Can you work these out from the model? Positions are in its coordinate system, mm. Give positions to 0.01 mm unless a question says otherwise; leave off trailing zeros. Loops run counter-clockwise (first coordinate to the right, second up) from the corner with the lowest first, then second, coordinate; pieces in that order, holes last. Notation, with made-up numbers: (4, 84.25) - (23, 84.25) arc R28 cw to (23, 120.25) - close; hole circle Ø1 at (56, -19). An arc over 180 degrees is marked (long way). Write item = value, one per line.
from build123d import *

# Parameters (mm, degrees)
SKETCH1_W          = 10.6426
SKETCH1_H          = 1.999996
SKETCH3_R          = 8.128
CUT_EXTRUDE1_DEPTH = 2.999996


with BuildPart() as part:
    # Sketch1 → Revolve1 (revolve)
    with BuildSketch(Plane.XY):
        with Locations((5.3213, 0)):
            Rectangle(SKETCH1_W, SKETCH1_H)
    revolve(axis=Axis((0, 0.999998, 0), (0, -1, 0)))

    # Sketch2 → Cut-Revolve1 (revolve, cut)
    with BuildSketch(Plane.XY):
        Polygon((-9.144, 0.635), (-9.144, 1.217425169), (-10.7442, 1.217425169), align=None)
        Polygon((-10.7442, -1.217425169), (-9.144, -0.635), (-9.144, -1.217425169), align=None)
    revolve(axis=Axis((0, 0, 0), (0, 1, 0)), mode=Mode.SUBTRACT)

    # Sketch3 → Cut-Extrude1 (cut, through all)
    with BuildSketch(Plane(origin=(0, 0.999998, 0), x_dir=(1, 0, 0), z_dir=(0, 1, 0))):
        Circle(SKETCH3_R)
    extrude(amount=-CUT_EXTRUDE1_DEPTH, mode=Mode.SUBTRACT)


solid = part.part
Q1. Imagine slicing it at A-A, the plane z = 0. Write out the boundary of the cut face in (x, y) (3 decimals), then the cut area to 3 significant figures.
Output:
outline = (-10.643, -1) - (-10.147, -1) - (-9.144, -0.635) - (-9.144, -1) - (-8.128, -1) - (-8.128, 1) - (-9.144, 1) - (-9.144, 0.635) - (-10.147, 1) - (-10.643, 1) - close; (8.128, -1) - (9.144, -1) - (9.144, -0.635) - (10.147, -1) - (10.643, -1) - (10.643, 1) - (10.147, 1) - (9.144, 0.635) - (9.144, 1) - (8.128, 1) - close
area = 9.33 mm2
Q2. For pin 1 (10 mm diameter, centred on x = 0, z = 0, fed in from +Y); pin 2 (4 mm diameter, centred on x = 5.5, z = -4.5, fed in from +Y), each with a flat end and sliding along its axis, tell me the tip position at first contact or that it passes through.
Output:
pin_1 = through
pin_2 = 1
Q3. I need wall thicknesses on L1, parallel to X at y = -0.15, z = 0.25; L2, parallel to Z at x = 0, y = 0.2; L3, parallel to X at y = 0.4, z = -6.5. Which ranges of each line are inside material? Lowest first, please.
Output:
L1 = -10.64 to -8.12, 8.12 to 10.64
L2 = -10.64 to -8.13, 8.13 to 10.64
L3 = -8.43 to -4.88, 4.88 to 8.43
Q4. We'd pull the mould along X, two halves only. Please class faces 1 (the cylindrical face through (1.982, -0.82, -8.927)), 2 (the flat face through (8.2, -1, -1.3)), 3 (the cylindrical face through (-2.31, 0.01, -10.39)): released by +X, released by -X, zero draft, split by the parting line, or undercut.
Output:
face_1 = undercut
face_2 = zero draft
face_3 = split by the parting line
Q5. Imagine slicing it at B-B, the plane x = 0. Write out the boundary of the cut face in (y, z) (3 decimals).
Output:
outline = (-1, -10.643) - (1, -10.643) - (1, -10.147) - (0.635, -9.144) - (1, -9.144) - (1, -8.128) - (-1, -8.128) - (-1, -9.144) - (-0.635, -9.144) - (-1, -10.147) - close; (-1, 8.128) - (1, 8.128) - (1, 9.144) - (0.635, 9.144) - (1, 10.147) - (1, 10.643) - (-1, 10.643) - (-1, 10.147) - (-0.635, 9.144) - (-1, 9.144) - close
Q6. Imagine slicing it at C-C, the plane y = 0.2. Write out the boundary of the cut face in (x, z), then the cut area to 3 significant figures.
Output:
outline = circle Ø21.29 at (0, 0); hole circle Ø16.26 at (0, 0)
area = 148 mm2
